Build history of the part. All positions in model axes, mm. Coordinates: 2 decimals unless noted, no trailing zeros. Loops run counter-clockwise (first coordinate to the right, second up) from the corner with the lowest first, then second, coordinate; pieces in that order, holes last. Notation, with made-up numbers: (29.5, 17.5) - (74.5, 17.5) arc R26 ccw to (74.5, 56.5) - close; hole circle Ø3 at (-29, -4.5). An arc over 180 degrees is marked (long way). One line per item, written item: value.
```python
from build123d import *

# Parameters (mm, degrees)
F1_DEPTH = 7


# Not quite as in the source:
# - a feature names something its author has since deleted; it is built from what else it names


with BuildPart() as f1:
    # F0 (on Top) → F1 (new body)
    with BuildSketch(Plane.XY):
        with BuildLine():
            ThreePointArc((0, 11), (7.7781745931, 7.7781745931), (11, 0))
            ThreePointArc((11, 0), (7.7781745931, -7.7781745931), (0, -11))
            Line((0, -11), (0, -16.5))
            ThreePointArc((0, -16.5), (11.6672618896, -11.6672618896), (16.5, 0))
            ThreePointArc((16.5, 0), (11.6672618896, 11.6672618896), (0, 16.5))
            Line((0, 16.5), (0, 11))
        make_face()
        with BuildLine():
            ThreePointArc((0, -11), (-11, 0), (0, 11))
            Line((0, 11), (0, 16.5))
            ThreePointArc((0, 16.5), (-11.6672618896, 11.6672618896), (-16.5, 0))
            ThreePointArc((-16.5, 0), (-11.6672618896, -11.6672618896), (0, -16.5))
            Line((0, -16.5), (0, -11))
        make_face()
        with BuildLine():
            Line((0, 19.5), (0, 16.5))
            ThreePointArc((0, 16.5), (11.6672618896, 11.6672618896), (16.5, 0))
            Line((16.5, 0), (16.5, 36))
            ThreePointArc((16.5, 36), (11.6672618896, 24.3327381104), (0, 19.5))
        make_face()
        with BuildLine():
            ThreePointArc((-16.5, 0), (-11.6672618896, 11.6672618896), (0, 16.5))
            Line((0, 16.5), (0, 19.5))
            ThreePointArc((0, 19.5), (-11.6672618896, 24.3327381104), (-16.5, 36))
            Line((-16.5, 36), (-16.5, 0))
        make_face()
        with BuildLine():
            Line((0, -19.5), (0, -16.5))
            ThreePointArc((0, -16.5), (-11.6672618896, -11.6672618896), (-16.5, 0))
            Line((-16.5, 0), (-16.5, -36))
            ThreePointArc((-16.5, -36), (-11.6672618896, -24.3327381104), (0, -19.5))
        make_face()
        with BuildLine():
            ThreePointArc((16.5, 0), (11.6672618896, -11.6672618896), (0, -16.5))
            Line((0, -16.5), (0, -19.5))
            ThreePointArc((0, -19.5), (11.6672618896, -24.3327381104), (16.5, -36))
            Line((16.5, -36), (16.5, 0))
        make_face()
        with BuildLine():
            ThreePointArc((-16.5, 36), (-11.6672618896, 24.3327381104), (0, 19.5))
            ThreePointArc((0, 19.5), (11.6672618896, 24.3327381104), (16.5, 36))
            ThreePointArc((16.5, 36), (0, 52.5), (-16.5, 36))
        make_face()
        with BuildLine():
            ThreePointArc((11, 36), (7.7781745931, 28.2218254069), (0, 25))
            ThreePointArc((0, 25), (-7.7781745931, 43.7781745931), (11, 36))
        make_face(mode=Mode.SUBTRACT)
        with BuildLine():
            ThreePointArc((16.5, -36), (11.6672618896, -24.3327381104), (0, -19.5))
            ThreePointArc((0, -19.5), (-11.6672618896, -24.3327381104), (-16.5, -36))
            ThreePointArc((-16.5, -36), (0, -52.5), (16.5, -36))
        make_face()
        with BuildLine():
            ThreePointArc((11, -36), (-7.7781745931, -43.7781745931), (0, -25))
            ThreePointArc((0, -25), (7.7781745931, -28.2218254069), (11, -36))
        make_face(mode=Mode.SUBTRACT)
    extrude(amount=F1_DEPTH)


solid = f1.part
```
Item 1: Cut at A-A, the plane y = -10. Write the cut outline in (x, z), then the cut area to 3 significant figures.
Check result:
outline: (-16.5, 0) - (-4.58, 0) - (-4.58, 7) - (-16.5, 7) - close; (4.58, 0) - (16.5, 0) - (16.5, 7) - (4.58, 7) - close
area: 167 mm^2
Item 2: Cut at C-C, the plane x = 8. Write the cut outline in (y, z).
Check result:
outline: (-50.43, 0) - (-43.55, 0) - (-43.55, 7) - (-50.43, 7) - close; (-28.45, 0) - (-7.55, 0) - (-7.55, 7) - (-28.45, 7) - close; (7.55, 0) - (28.45, 0) - (28.45, 7) - (7.55, 7) - close; (43.55, 0) - (50.43, 0) - (50.43, 7) - (43.55, 7) - close
Item 3: Probe probe 1 along X at (y, z) = (-36, 5.25); probe 2 along Y at (x, z) = (2, 0.5); probe 3 along Y at (x, z) = (9.5, 4.25). List the from-to ranges inside material, lowest first. Write a range as from..to.
Check result:
probe 1: x = -16.5..-11, 11..16.5
probe 2: y = -52.38..-46.82, -25.18..-10.82, 10.82..25.18, 46.82..52.38
probe 3: y = -49.49..-41.55, -30.45..-5.55, 5.55..30.45, 41.55..49.49
Item 4: Drop a flat-ended pin along its axis: P1, Ø2, axis at x = -9.5, y = 34.5, coming from the +Z side. Give the stop position or say it passes through.
Check result:
P1: passes through
Item 5: Cut at D-D, the plane y = -31. Write the cut outline in (x, z).
Check result:
outline: (-16.5, 0) - (-9.8, 0) - (-9.8, 7) - (-16.5, 7) - close; (9.8, 0) - (16.5, 0) - (16.5, 7) - (9.8, 7) - close
Item 6: Cut at B-B, the plane z = 2.5. Write the cut outline in (x, y).
Check result:
outline: (-16.5, -36) arc R16.5 ccw to (16.5, -36) - (16.5, 36) arc R16.5 ccw to (-16.5, 36) - close; hole circle Ø22 at (0, -36); hole circle Ø22 at (0, 0); hole circle Ø22 at (0, 36)
